Here's how the part is built. I have some questions about the finished solid (model axes, mm). A direction names the side the tool comes from. Give positions to 0.01 mm unless a question says otherwise; leave off trailing zeros. Order: outer loops, then holes, each group sorted by start corner. A loop starts at its lowest first (then second) coordinate and runs counter-clockwise, first axis right, second up.
from build123d import *

# Parameters (mm, degrees)
BOSS_EXTRUDE2_DEPTH = 40
SKETCH3_R           = 4.05
CUT_EXTRUDE1_DEPTH  = 35
CUT_EXTRUDE2_REACH  = 19
SKETCH4_R           = 3.25
SKETCH6_R           = 1.5
CUT_EXTRUDE3_DEPTH  = 10


with BuildPart() as part:
    # Sketch1 → Boss-Extrude2 (new body)
    with BuildSketch(Plane(origin=(0, 0, 0), x_dir=(1, 0, 0), z_dir=(0, 1, 0))):
        Polygon((-10, -5.257459708), (-10, 0.742540292), (10, 0.742540292), (10, -5.257459708), (25, -5.257459708), (25, -22.257459708), (-10, -22.257459708), align=None)
    extrude(amount=BOSS_EXTRUDE2_DEPTH)

    # Sketch3 → Cut-Extrude1 (cut)
    with BuildSketch(Plane.XZ):
        with Locations((0, 7.257459708)):
            Circle(SKETCH3_R)
    extrude(amount=-CUT_EXTRUDE1_DEPTH, mode=Mode.SUBTRACT)

    # Sketch4 → Cut-Extrude2 (cut, up to next)
    with BuildSketch(Plane(origin=(0, 0, 5.257459708), x_dir=(-1, 0, 0), z_dir=(0, 0, -1)), mode=Mode.PRIVATE) as cut_extrude2_sk1:
        with Locations((-17.5, 26.045770547)):
            Circle(SKETCH4_R)
    cut_extrude2_tool1 = extrude(cut_extrude2_sk1.sketch, amount=-CUT_EXTRUDE2_REACH, mode=Mode.PRIVATE) & part.part
    add(cut_extrude2_tool1.solids().sort_by_distance((17.5, 26.045771, 5.25746))[0], mode=Mode.SUBTRACT)
    # Sketch4 → Cut-Extrude2 (cut, up to next)
    with BuildSketch(Plane(origin=(0, 0, 5.257459708), x_dir=(-1, 0, 0), z_dir=(0, 0, -1)), mode=Mode.PRIVATE) as cut_extrude2_sk2:
        with Locations((-17.5, 7.535290978)):
            Circle(SKETCH4_R)
    cut_extrude2_tool2 = extrude(cut_extrude2_sk2.sketch, amount=-CUT_EXTRUDE2_REACH, mode=Mode.PRIVATE) & part.part
    add(cut_extrude2_tool2.solids().sort_by_distance((17.5, 7.535291, 5.25746))[0], mode=Mode.SUBTRACT)

    # Sketch6 → Cut-Extrude3 (cut)
    with BuildSketch(Plane.XZ.offset(-35)):
        with Locations((0, 7.257459708)):
            Circle(SKETCH6_R)
    extrude(amount=-CUT_EXTRUDE3_DEPTH, mode=Mode.SUBTRACT)


with BuildPart() as body_2:
    # Mirror4: mirrored copy
    add(part.part.mirror(Plane.ZX))


solid = body_2.part
Q1. If we section it at D-D on x = 0: List the corners of the cut face in (y, z) for me.
Filled sheet:
outline: (-40, -0.74) - (0, -0.74) - (0, 3.21) - (-35, 3.21) - (-35, 5.76) - (-40, 5.76) - close; (-40, 8.76) - (-35, 8.76) - (-35, 11.31) - (0, 11.31) - (0, 22.26) - (-40, 22.26) - close
Q2. If we section it at A-A on z = 6.75: List the corners of the cut face in (x, y) for me.
Filled sheet:
outline: (-10, -40) - (-1.41, -40) - (-1.41, -35) - (-4.02, -35) - (-4.02, 0) - (-10, 0) - close; (1.41, -40) - (25, -40) - (25, 0) - (4.02, 0) - (4.02, -35) - (1.41, -35) - close; hole circle Ø6.5 at (17.5, -26.05); hole circle Ø6.5 at (17.5, -7.54)
Q3. If we section it at C-C on y = -9: List the corners of the cut face in (x, z) for me, plus the area to 3 significant figures.
Filled sheet:
outline: (-10, -0.74) - (10, -0.74) - (10, 5.26) - (14.6, 5.26) - (14.6, 22.26) - (-10, 22.26) - close; (20.4, 5.26) - (25, 5.26) - (25, 22.26) - (20.4, 22.26) - close; hole circle Ø8.1 at (0, 7.26)
area: 565 mm2
Q4. I'm going to push flat-ended pins straight in: P1, Ø4, axis at x = 0, z = 7.26, coming from the +Y side; P2, Ø1.5, axis at x = 14.5, y = -21, coming from the -Z side; P3, Ø3, axis at y = -29.5, z = 2.5, coming from the +X side. Where does each tip first touch, or does it pass through?
Filled sheet:
P1: stops at y = -35
P2: stops at z = 5.26
P3: stops at x = 10
Q5. Thinking about a two-plate mould opening in X: for faces 1 (the face through (8, -20, 22.257)), 2 (the face through (-0.1, -35, 5.5)), 3 (the face through (25, -20, 14)), 4 (the face through (20.08, -24.07, 13.64)), which applies, released by +X, released by -X, zero draft, split by the parting line, or undercut?
Filled sheet:
face 1: zero draft
face 2: undercut
face 3: released by +X
face 4: undercut
Q6. I need wall thicknesses on L1, parallel to Y at x = 17.5, z = 13.5; L2, parallel to Y at x = 17, z = 16.75; L3, parallel to X at y = -26.5, z = 9.75. Which ranges of each line are inside material? Lowest first, please.
Filled sheet:
L1: y = -40 to -29.3, -22.8 to -10.79, -4.29 to 0
L2: y = -40 to -29.26, -22.83 to -10.75, -4.32 to 0
L3: x = -10 to -3.19, 3.19 to 14.28, 20.72 to 25
Q7. For faces 5 (the face through (10, -20, 2)), 6 (the face through (-0.527, -17.255, 11.273)), 7 (the face through (8, 0, 11)), which set-ups out of +Z, -Z, +X, -X, +Y, -Y let a thin tool reach every point of the face, with its end or its side?
Filled sheet:
face 5: -Z, +X, +Y, -Y
face 6: +Y
face 7: +Z, -Z, +X, -X, +Y
Q8. If we section it at B-B on x = 17.5: List the corners of the cut face in (y, z) for me, plus the area to 3 significant figures.
Filled sheet:
outline: (-40, 5.26) - (-29.3, 5.26) - (-29.3, 22.26) - (-40, 22.26) - close; (-22.8, 5.26) - (-10.79, 5.26) - (-10.79, 22.26) - (-22.8, 22.26) - close; (-4.29, 5.26) - (0, 5.26) - (0, 22.26) - (-4.29, 22.26) - close
area: 459 mm2
